from build123d import *

# Parameters (mm, degrees)
SKETCH1_W                = 80
SKETCH1_H                = 45
SKETCH1_R                = 13
SKETCH1_R_2              = 2.075
BOSS_EXTRUDE1_DEPTH      = 5
BOSS_EXTRUDE2_DEPTH      = 150
BOSS_EXTRUDE2_DEPTH_BACK = 5
SKETCH2_W                = 80
SKETCH2_H                = 5
FILLET1_R                = 4
FILLET2_R                = 1


with BuildPart() as part:
    # Sketch1 → Boss-Extrude1 (new body)
    with BuildSketch(Plane.XY):
        Rectangle(SKETCH1_W, SKETCH1_H)
        Circle(SKETCH1_R, mode=Mode.SUBTRACT)
        with Locations((0, 17.5)):
            Circle(SKETCH1_R_2, mode=Mode.SUBTRACT)
        with Locations((17.5, 0)):
            Circle(SKETCH1_R_2, mode=Mode.SUBTRACT)
        with Locations((0, -17.5)):
            Circle(SKETCH1_R_2, mode=Mode.SUBTRACT)
        with Locations((-17.5, 0)):
            Circle(SKETCH1_R_2, mode=Mode.SUBTRACT)
    extrude(amount=BOSS_EXTRUDE1_DEPTH)

    # Sketch2 → Boss-Extrude2 (add, two sides: drawn at the far end of the back side and taken through both)
    with BuildSketch(Plane(origin=(0, 0, 0), x_dir=(-1, 0, 0), z_dir=(0, 0, -1)).offset(-BOSS_EXTRUDE2_DEPTH_BACK)):
        with Locations((0, -25)):
            Rectangle(SKETCH2_W, SKETCH2_H)
    extrude(amount=BOSS_EXTRUDE2_DEPTH + BOSS_EXTRUDE2_DEPTH_BACK)

    # Fillet1
    fillet1_edges = [part.edges().sort_by_distance(p)[0] for p in [
        (0, -27.5, 5),
        (40, -25, -150),
        (-40, -25, -150),
        (-40, 22.5, 2.5),
        (40, 22.5, 2.5),
    ]]
    fillet(fillet1_edges, radius=FILLET1_R)

    # Fillet2
    fillet2_edges = [part.edges().sort_by_distance(p)[0] for p in [
        (0, -22.5, 0),
    ]]
    fillet(fillet2_edges, radius=FILLET2_R)


solid = part.part
For this review, take the finished solid that the model builds, in its own axes (mm). A direction names the side the tool comes from. Coordinates: 2 decimals unless noted, no trailing zeros. Loops run counter-clockwise (first coordinate to the right, second up) from the corner with the lowest first, then second, coordinate; pieces in that order, holes last. Notation, with made-up numbers: (18.5, 58) - (68.5, 58) arc R23 ccw to (68.5, 86) - close; hole circle Ø1 at (50, 0.5). An arc over 180 degrees is marked (long way). Use a Markdown table: item, result. Add a question column.
Item 1: Tool access review of faces 4 (the face through (-0.56, -26.297, 3.859)), 5 (the face through (-9, 11, 0)): name each direction out of +Z, -Z, +X, -X, +Y, -Y from which nothing blocks a thin tool from reaching the whole face with its end or side.
Item 2: We need section B-B (y = 0). Give the boundary of the cut face in (x, z) (3 decimals), and give its area (4 significant figures).
Item 3: For line 1 (Y direction, x = 0, z = 2.85) (3 decimals); line 2 (Y direction, x = 0, z = 3.5) (1 decimal); line 3 (Y direction, x = 30.5, z = -143), list the stretches that pass through material, from the lowest coordinate up.
Item 4: We need section A-A (x = -17.5). Give the boundary of the cut face in (y, z) (3 decimals).
Item 5: Mouldability with a two-part tool opening along Y and no side actions: class faces 1 (the face through (1, -27.5, -73)), 2 (the face through (19.48, 0.62, 2.46)), 3 (the face through (-38.859, 21.297, 2.535)) as pulls with the +Y half, pulls with the -Y half, needs draft (parallel to the pull), parting line crosses it, or undercut.
Item 6: We need section C-C (x = 0). Give the boundary of the cut face in (y, z) (3 decimals), and give its area (3 significant figures).
Item 7: We need section D-D (y = -17.5). Give the boundary of the cut face in (x, z) (3 decimals).
Item 8: Insertion check: pin 1 Ø5.5 at (x, y) = (-17.5, 0) entering from -Z; pin 2 Ø6 at (x, z) = (-8, -13) entering from +Y. Each pin has a flat end and moves straight along its axis. Give the tip position at first contact, or say it passes through.
Results list:
| question | item | result |
|---|---|---|
| 1 | face 4 | +Z, +X, -X, -Y |
| 1 | face 5 | -Z, +X, -X, +Y |
| 2 | outline | (-40, 0) - (-19.575, 0) - (-19.575, 5) - (-40, 5) - close; (-15.425, 0) - (-13, 0) - (-13, 5) - (-15.425, 5) - close; (13, 0) - (15.425, 0) - (15.425, 5) - (13, 5) - close; (19.575, 0) - (40, 0) - (40, 5) - (19.575, 5) - close |
| 2 | area | 228.5 mm^2 |
| 3 | line 1 | y = -27.046 to -19.575, -15.425 to -13, 13 to 15.425, 19.575 to 22.5 |
| 3 | line 2 | y = -26.6 to -19.6, -15.4 to -13, 13 to 15.4, 19.6 to 22.5 |
| 3 | line 3 | y = -27.5 to -22.5 |
| 4 | outline | (-27.5, -150) - (-22.5, -150) - (-22.5, -1) arc R1 cw to (-21.5, 0) - (-2.075, 0) - (-2.075, 5) - (-23.5, 5) arc R4 ccw to (-27.5, 1) - close; (2.075, 0) - (22.5, 0) - (22.5, 5) - (2.075, 5) - close |
| 5 | face 1 | pulls with the -Y half |
| 5 | face 2 | undercut |
| 5 | face 3 | pulls with the +Y half |
| 6 | outline | (-27.5, -150) - (-22.5, -150) - (-22.5, -1) arc R1 cw to (-21.5, 0) - (-19.575, 0) - (-19.575, 5) - (-23.5, 5) arc R4 ccw to (-27.5, 1) - close; (-15.425, 0) - (-13, 0) - (-13, 5) - (-15.425, 5) - close; (13, 0) - (15.425, 0) - (15.425, 5) - (13, 5) - close; (19.575, 0) - (22.5, 0) - (22.5, 5) - (19.575, 5) - close |
| 6 | area | 825 mm^2 |
| 7 | outline | (-40, 0) - (-2.075, 0) - (-2.075, 5) - (-40, 5) - close; (2.075, 0) - (40, 0) - (40, 5) - (2.075, 5) - close |
| 8 | pin 1 | stops at z = 0 |
| 8 | pin 2 | stops at y = -22.5 |
